```python
from build123d import *

# Parameters (mm, degrees)
SKETCH_R     = 2.8
PAD_DEPTH    = 3
SKETCH001_R  = 1.45
PAD001_DEPTH = 20
POCKET_DEPTH = 2
CHAMFER_SIZE = 0.25


with BuildPart() as part:
    # Sketch → Pad (new body)
    with BuildSketch(Plane.XY):
        Circle(SKETCH_R)
    extrude(amount=PAD_DEPTH)

    # Sketch001 (on Face3 of Pad) → Pad001 (join)
    with BuildSketch(Plane.XY.offset(3)):
        Circle(SKETCH001_R)
    extrude(amount=PAD001_DEPTH)

    # Sketch002 (on Face2 of Pad001) → Pocket (cut)
    with BuildSketch(Plane(origin=(0, 0, 0), x_dir=(1, 0, 0), z_dir=(0, 0, -1))):
        Polygon((1.259542, 0.814588), (-0.075682, 1.49809), (-1.335225, 0.683502), (-1.259542, -0.814588), (0.075682, -1.49809), (1.335225, -0.683502), align=None)
    extrude(amount=-POCKET_DEPTH, mode=Mode.SUBTRACT)

    # Chamfer
    chamfer_edges = [part.edges().sort_by_distance(p)[0] for p in [
        (-2.8, 0, 3),
        (-2.8, 0, 0),
        (1.297384, -0.065543, 0),
        (0.705454, 1.090796, 0),
        (-0.59193, 1.156339, 0),
        (-1.297384, 0.065543, 0),
        (-0.705454, -1.090796, 0),
        (0.59193, -1.156339, 0),
        (-1.45, 0, 23),
    ]]
    chamfer(chamfer_edges, length=CHAMFER_SIZE)


solid = part.part
```
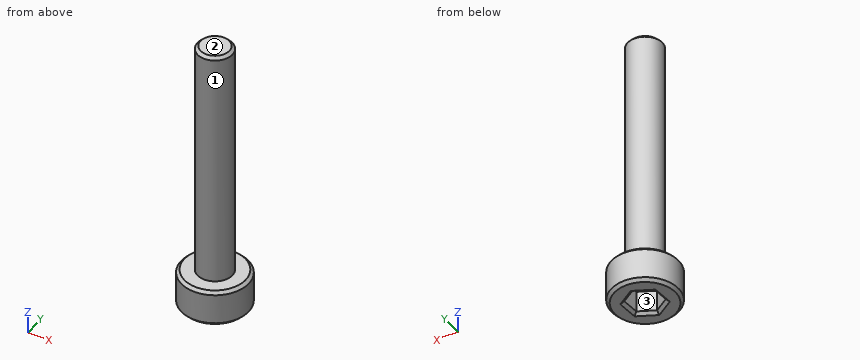
Geometry check sheet. Reference: the model listing, model coordinates, mm. Face numbers are marked on the shaded views. Coordinates: 2 decimals unless noted, no trailing zeros. Order: outer loops, then holes, each group sorted by start corner. A loop starts at its lowest first (then second) coordinate and runs counter-clockwise, first axis right, second up.
Q1. Sectioned sample at A-A on y = 0. Record the cut outline in (x, z).
Reply:
outline: (-2.8, 0.25) - (-2.55, 0) - (-1.55, 0) - (-1.3, 0.25) - (-1.3, 2) - (1.3, 2) - (1.3, 0.25) - (1.55, 0) - (2.55, 0) - (2.8, 0.25) - (2.8, 2.75) - (2.55, 3) - (1.45, 3) - (1.45, 22.75) - (1.2, 23) - (-1.2, 23) - (-1.45, 22.75) - (-1.45, 3) - (-2.55, 3) - (-2.8, 2.75) - close
Q2. Depth check by flat-ended pin: pin 1 Ø1.5 at (x, z) = (-1, 6.5) entering from +Y; pin 2 Ø0.8 at (x, y) = (0.5, 0) entering from -Z; pin 3 Ø1.5 at (x, z) = (-1.5, 12) entering from -Y. Enter the tip coordinate at first touch or a pass-through.
Reply:
pin 1: stops at y = 1.43
pin 2: stops at z = 2
pin 3: stops at y = -1.24
Q3. Sectioned sample at C-C on z = 11.75. Record the cut outline in (x, y).
Reply:
outline: circle Ø2.9 at (0, 0)
Q4. Thickness scan on probe 1 along Y at (x, z) = (-0.1, 19.25); probe 2 along Z at (x, y) = (1.6, -1.45); probe 3 along Z at (x, y) = (-0.1, 0.05). Record the ranges inside material, lowest first.
Reply:
probe 1: y = -1.45 to 1.45
probe 2: z = 0 to 3
probe 3: z = 2 to 23
Q5. Draft check along Y on the marked faces 1, 2 and 3. Enter one of: released by +Y, released by -Y, zero draft, split by the parting line, or undercut.
Reply:
face 1: split by the parting line
face 2: zero draft
face 3: undercut
Q6. Sectioned sample at B-B on z = 2.5. Record the cut outline in (x, y).
Reply:
outline: circle Ø5.6 at (0, 0)
